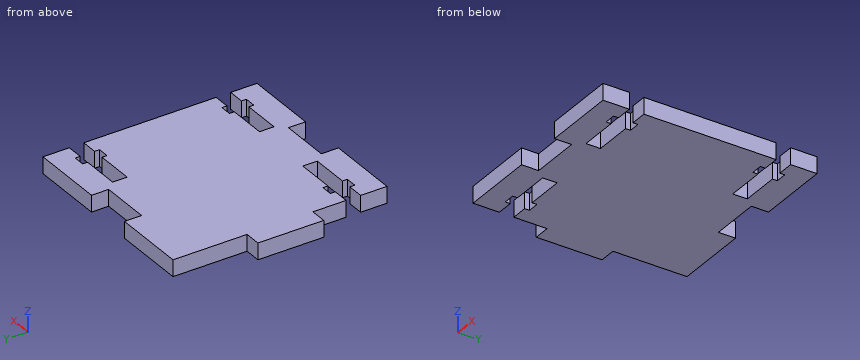
from build123d import *

# Parameters (mm, degrees)
BOSS_EXTRUDE1_DEPTH = 5
CUT_EXTRUDE1_DEPTH  = 5
SKETCH4_W           = 15.2
SKETCH4_H           = 5.2
CUT_EXTRUDE2_DEPTH  = 10


with BuildPart() as part:
    # Sketch1 → Boss-Extrude1 (new body)
    with BuildSketch(Plane.XY):
        Polygon((-30, 32.5), (-7.5, 32.5), (30, 32.5), (30, -32.5), (-30, -32.5), (-30, -10), (-35, -10), (-35, 10), (-30, 10), align=None)
    extrude(amount=BOSS_EXTRUDE1_DEPTH)

    # Sketch3 → Cut-Extrude1 (cut)
    with BuildSketch(Plane.XY.offset(5)):
        Polygon((30, 24.5), (25, 24.5), (25, 26), (21.6, 26), (21.6, 24.5), (10, 24.5), (10, 20.1), (21.6, 20.1), (21.6, 18.6), (25, 18.6), (25, 20.1), (30, 20.1), align=None)
        Polygon((30, -24.5), (30, -20.1), (25, -20.1), (25, -18.6), (21.6, -18.6), (21.6, -20.1), (10, -20.1), (10, -24.5), (21.6, -24.5), (21.6, -26), (25, -26), (25, -24.5), align=None)
        Polygon((-30, -24.5), (-25, -24.5), (-25, -26), (-21.6, -26), (-21.6, -24.5), (-10, -24.5), (-10, -20.1), (-21.6, -20.1), (-21.6, -18.6), (-25, -18.6), (-25, -20.1), (-30, -20.1), align=None)
    extrude(amount=-CUT_EXTRUDE1_DEPTH, mode=Mode.SUBTRACT)

    # Sketch4 → Cut-Extrude2 (cut)
    with BuildSketch(Plane.XY.offset(5)):
        with Locations((0, -29.9)):
            Rectangle(SKETCH4_W, SKETCH4_H)
        with Locations((0, 29.9)):
            Rectangle(SKETCH4_W, SKETCH4_H)
    extrude(amount=-CUT_EXTRUDE2_DEPTH, mode=Mode.SUBTRACT)


solid = part.part
Input: part model. Units: mm. Frame: model coordinates. Coordinates: 2 decimals unless noted, no trailing zeros. Loops run counter-clockwise (first coordinate to the right, second up) from the corner with the lowest first, then second, coordinate; pieces in that order, holes last.
(1) Section A-A on x = -23.5. Return the cut outline in (y, z), then the cut area to 3 significant figures.
(2) Section C-C on y = 14. Return the cut outline in (x, z), then the cut area to 3 significant figures.
(3) Section B-B on x = 15. Return the cut outline in (y, z).
(4) Section D-D on x = -4. Return the cut outline in (y, z).
(5) First-contact query: pin 1 Ø2.5 at (y, z) = (-30, 1.5) entering from -X; pin 2 Ø1.5 at (x, z) = (-2, 3) entering from -Y; pin 3 Ø2 at (x, y) = (20, -17.5) entering from -Z. Flat tips, straight axial feed; report the tip coordinate or a pass-through.
(6) Material intervals for probe 1 along Y at (x, z) = (20.5, 2.5); probe 2 along Y at (x, z) = (24, 0.6); probe 3 along X at (y, z) = (-25.5, 3.2), sorted ascending.
Data:
1. outline: (-32.5, 0) - (-26, 0) - (-26, 5) - (-32.5, 5) - close; (-18.6, 0) - (32.5, 0) - (32.5, 5) - (-18.6, 5) - close
1. area: 288 mm2
2. outline: (-30, 0) - (30, 0) - (30, 5) - (-30, 5) - close
2. area: 300 mm2
3. outline: (-32.5, 0) - (-24.5, 0) - (-24.5, 5) - (-32.5, 5) - close; (-20.1, 0) - (20.1, 0) - (20.1, 5) - (-20.1, 5) - close; (24.5, 0) - (32.5, 0) - (32.5, 5) - (24.5, 5) - close
4. outline: (-27.3, 0) - (27.3, 0) - (27.3, 5) - (-27.3, 5) - close
5. pin 1: stops at x = -30
5. pin 2: stops at y = -27.3
5. pin 3: stops at z = 0
6. probe 1: y = -32.5 to -24.5, -20.1 to 20.1, 24.5 to 32.5
6. probe 2: y = -32.5 to -26, -18.6 to 18.6, 26 to 32.5
6. probe 3: x = -30 to -25, -21.6 to 21.6, 25 to 30
